from build123d import *
from build123d.topology import SkipClean

# Parameters (mm, degrees)
BOSS_EXTRUDE1_DEPTH = 11
SKETCH3_R           = 2.9
SKETCH3_R_2         = 0.5
CUT_EXTRUDE1_DEPTH  = 4
SKETCH4_W           = 15.75
SKETCH4_H           = 9.4
BOSS_EXTRUDE2_DEPTH = 1
SKETCH5_W           = 15.75
SKETCH5_H           = 9.4
SKETCH5_R           = 1.85
SKETCH5_R_2         = 2.8
CUT_EXTRUDE2_DEPTH  = 1
SKETCH6_W           = 15.75
SKETCH6_H           = 9.4
BOSS_EXTRUDE3_DEPTH = 0.3
CUT_EXTRUDE3_DEPTH  = 0.2
CUT_EXTRUDE4_DEPTH  = 0.1


with BuildPart() as part:
    # Sketch1 → Boss-Extrude1 (new body)
    with BuildSketch(Plane.XY):
        with BuildLine():
            Line((-3, 26.502943725), (-3, -1.102943725))
            ThreePointArc((-3, -1.102943725), (-2.908655439, -1.562163844), (-2.648528137, -1.951471863))
            Line((-2.648528137, -1.951471863), (-2.151471863, -2.448528137))
            ThreePointArc((-2.151471863, -2.448528137), (-1.762163844, -2.708655439), (-1.302943725, -2.8))
            Line((-1.302943725, -2.8), (10.002943725, -2.8))
            ThreePointArc((10.002943725, -2.8), (10.462163844, -2.708655439), (10.851471863, -2.448528137))
            Line((10.851471863, -2.448528137), (16.648528137, 3.348528137))
            ThreePointArc((16.648528137, 3.348528137), (16.908655439, 3.737836156), (17, 4.197056275))
            Line((17, 4.197056275), (17, 27))
            ThreePointArc((17, 27), (16.648528137, 27.848528137), (15.8, 28.2))
            Line((15.8, 28.2), (-1.302943725, 28.2))
            ThreePointArc((-1.302943725, 28.2), (-1.762163844, 28.108655439), (-2.151471863, 27.848528137))
            Line((-2.151471863, 27.848528137), (-2.648528137, 27.351471863))
            ThreePointArc((-2.648528137, 27.351471863), (-2.908655439, 26.962163844), (-3, 26.502943725))
        make_face()
    extrude(amount=-BOSS_EXTRUDE1_DEPTH)

    # Sketch2 → Revolve1 (revolve)
    with BuildSketch(Plane.XY.offset(-5.5), mode=Mode.PRIVATE) as revolve1_sk:
        with BuildLine():
            Line((12, 4.7), (16.899094141, 4.7))
            Line((16.899094141, 4.7), (15.897307991, -4.831358539))
            ThreePointArc((15.897307991, -4.831358539), (15.799690604, -5.022943448), (15.598951422, -5.1))
            Line((15.598951422, -5.1), (15.45, -5.1))
            Line((15.45, -5.1), (15.45, -6.1))
            Line((15.45, -6.1), (16, -6.1))
            Line((16, -6.1), (16, -10.1))
            Line((16, -10.1), (15.25, -10.1))
            Line((15.25, -10.1), (15.25, -11.6))
            Line((15.25, -11.6), (15.45, -11.6))
            Line((15.45, -11.6), (15.45, -12.1))
            Line((15.45, -12.1), (15.25, -13.1))
            Line((15.25, -13.1), (12, -13.1))
            Line((12, -13.1), (12, 4.7))
        make_face()
    revolve(revolve1_sk.sketch.rotate(Axis((12, -13.1, -5.5), (0, 1, 0)), 270), axis=Axis((12, -13.1, -5.5), (0, 1, 0)))

    # Sketch3 → Cut-Extrude1 (cut)
    with BuildSketch(Plane(origin=(0, -9.3, 0), x_dir=(1, 0, 0), z_dir=(0, 1, 0))):
        with Locations(Location((12, 5.5, 0), (0, 0, 270))):
            Circle(SKETCH3_R)
        with Locations(Location((13.41577974, 4.471375808, 0), (0, 0, 270))):
            Circle(SKETCH3_R_2, mode=Mode.SUBTRACT)
        with Locations(Location((13.41577974, 6.528624192, 0), (0, 0, 270))):
            Circle(SKETCH3_R_2, mode=Mode.SUBTRACT)
        with Locations(Location((11.45922026, 3.835651096, 0), (0, 0, 270))):
            Circle(SKETCH3_R_2, mode=Mode.SUBTRACT)
        with Locations(Location((11.45922026, 7.164348904, 0), (0, 0, 270))):
            Circle(SKETCH3_R_2, mode=Mode.SUBTRACT)
    extrude(amount=-CUT_EXTRUDE1_DEPTH, mode=Mode.SUBTRACT)

    # Sketch4 → Boss-Extrude2 (add)
    with BuildSketch(Plane(origin=(0, 28.2, 0), x_dir=(1, 0, 0), z_dir=(0, 1, 0))):
        with Locations((8.075, 5.5)):
            Rectangle(SKETCH4_W, SKETCH4_H)
        Polygon((11.656497116, 4.356497116), (12.529289322, 4.356497116), (12.305025253, 4.580761184), (13.789949494, 6.065685425), (13.365685425, 6.489949494), (11.880761184, 5.005025253), (11.656497116, 5.229289322), align=None, mode=Mode.SUBTRACT)
        Polygon((5.85, 5.9), (5.85, 5.1), (7.35, 5.1), (7.35, 3.6), (8.15, 3.6), (8.15, 5.1), (9.65, 5.1), (9.65, 5.9), (8.15, 5.9), (8.15, 7.4), (7.35, 7.4), (7.35, 5.9), align=None, mode=Mode.SUBTRACT)
    extrude(amount=BOSS_EXTRUDE2_DEPTH)

    # Sketch5 → Cut-Extrude2 (cut)
    with BuildSketch(Plane(origin=(0, 28.2, 0), x_dir=(1, 0, 0), z_dir=(0, 1, 0))):
        with Locations((8.075, 5.5)):
            Rectangle(SKETCH5_W, SKETCH5_H)
        with Locations(Location((12.8, 5.5, 0), (0, 0, 270))):
            Circle(SKETCH5_R, mode=Mode.SUBTRACT)
        with Locations(Location((7.75, 5.5, 0), (0, 0, 270))):
            Circle(SKETCH5_R_2, mode=Mode.SUBTRACT)
    extrude(amount=CUT_EXTRUDE2_DEPTH, mode=Mode.SUBTRACT)

    # Sketch6 → Boss-Extrude3 (add)
    with BuildSketch(Plane(origin=(0, 28.2, 0), x_dir=(1, 0, 0), z_dir=(0, 1, 0))):
        with Locations((8.075, 5.5)):
            Rectangle(SKETCH6_W, SKETCH6_H)
    extrude(amount=BOSS_EXTRUDE3_DEPTH)

    # Sketch7 → Revolve2 (revolve)
    with SkipClean():  # the faces are left unmerged after this step: merging them gives an invalid solid
        with BuildSketch(Plane(origin=(3.1, 0, 0), x_dir=(0, 0, -1), z_dir=(1, 0, 0))):
            with BuildLine():
                Line((8.85, 28), (5.75, 28))
                ThreePointArc((5.75, 28), (7.3, 29.55), (8.85, 28))
            make_face()
        revolve(axis=Axis((3.1, 28, -8.85), (0, 0, 1)))

    # Sketch8 → Cut-Extrude3 (cut)
    with SkipClean():  # the faces are left unmerged after this step: merging them gives an invalid solid
        with BuildSketch(Plane(origin=(-2.8, 0, 0), x_dir=(0, 0, -1), z_dir=(1, 0, 0))):
            with BuildLine():
                Line((1.425, 19.925), (1.425, 2.675))
                ThreePointArc((1.425, 2.675), (1.659314575, 2.109314575), (2.225, 1.875))
                Line((2.225, 1.875), (8.775, 1.875))
                ThreePointArc((8.775, 1.875), (9.340685425, 2.109314575), (9.575, 2.675))
                Line((9.575, 2.675), (9.575, 19.925))
                ThreePointArc((9.575, 19.925), (9.340685425, 20.490685425), (8.775, 20.725))
                Line((8.775, 20.725), (2.225, 20.725))
                ThreePointArc((2.225, 20.725), (1.659314575, 20.490685425), (1.425, 19.925))
            make_face()
        extrude(amount=-CUT_EXTRUDE3_DEPTH, mode=Mode.SUBTRACT)

    # Sketch9 → Cut-Extrude4 (cut)
    with SkipClean():  # the faces are left unmerged after this step: merging them gives an invalid solid
        with BuildSketch(Plane.XY.offset(-11)):
            with BuildLine():
                Line((4.4, 0.2), (9.091673888, 0.2))
                ThreePointArc((9.091673888, 0.2), (9.244747261, 0.230448187), (9.3745166, 0.317157288))
                Line((9.3745166, 0.317157288), (13.882842712, 4.8254834))
                ThreePointArc((13.882842712, 4.8254834), (13.969551813, 4.955252739), (14, 5.108326112))
                Line((14, 5.108326112), (14, 24.8))
                ThreePointArc((14, 24.8), (13.882842712, 25.082842712), (13.6, 25.2))
                Line((13.6, 25.2), (4.4, 25.2))
                ThreePointArc((4.4, 25.2), (4.117157288, 25.082842712), (4, 24.8))
                Line((4, 24.8), (4, 0.6))
                ThreePointArc((4, 0.6), (4.117157288, 0.317157288), (4.4, 0.2))
            make_face()
        extrude(amount=CUT_EXTRUDE4_DEPTH, mode=Mode.SUBTRACT)

    # Sketch10 → Cut-Revolve1 (revolve, cut)
    with SkipClean():  # the faces are left unmerged after this step: merging them gives an invalid solid
        with BuildSketch(Plane(origin=(0, 0, 0), x_dir=(0, 0, -1), z_dir=(1, 0, 0)), mode=Mode.PRIVATE) as cut_revolve1_sk:
            Polygon((0, 0), (0, 1.5), (0.2705, 1.2295), (10.7295, 1.2295), (11, 1.5), (11, 0), align=None)
        revolve(cut_revolve1_sk.sketch.rotate(Axis((0, 0, -11), (0, 0, 1)), 270), axis=Axis((0, 0, -11), (0, 0, 1)), mode=Mode.SUBTRACT)

    # Sketch11 → Cut-Revolve2 (revolve, cut)
    with SkipClean():  # the faces are left unmerged after this step: merging them gives an invalid solid
        with BuildSketch(Plane(origin=(0, 0, 0), x_dir=(0, 0, -1), z_dir=(1, 0, 0)), mode=Mode.PRIVATE) as cut_revolve2_sk:
            Polygon((0, 25.4), (0, 26.9), (0.2705, 26.6295), (10.7295, 26.6295), (11, 26.9), (11, 25.4), align=None)
        revolve(cut_revolve2_sk.sketch.rotate(Axis((0, 25.4, -11), (0, 0, 1)), 270), axis=Axis((0, 25.4, -11), (0, 0, 1)), mode=Mode.SUBTRACT)

    # Sketch12 → Revolve3 (revolve)
    with SkipClean():  # the faces are left unmerged after this step: merging them gives an invalid solid
        with BuildSketch(Plane(origin=(3.1, 0, 0), x_dir=(0, 0, -1), z_dir=(1, 0, 0))):
            with BuildLine():
                Line((5.15, 28), (2.05, 28))
                ThreePointArc((2.05, 28), (3.6, 29.55), (5.15, 28))
            make_face()
        revolve(axis=Axis((3.1, 28, -5.15), (0, 0, 1)))


solid = part.part
For this review, take the finished solid that the model builds, in its own axes (mm). A direction names the side the tool comes from. Round coordinates to 2 decimals unless told otherwise and drop trailing zeros. Write each question's results on one line, items separated by ' | '. Start each with the question number.
1. Draft analysis for pull direction X (two halves, no side actions). For faces 1 (the face through (13.44, -11.17, -4.97)), 2 (the face through (8.3, 29.2, -4.9)), 3 (the face through (5.266, 28.845, -4.208)), 4 (the face through (-2.91, -1.56, -5.42)), state which applies: pulls with the +X half, pulls with the -X half, needs draft (parallel to the pull), parting line crosses it, or undercut.
2. Clearance check with flat-ended pins moving along their axes: pin 1 Ø1.5 at (y, z) = (16, -4.5) entering from -X; pin 2 Ø5 at (y, z) = (-2.5, -7) entering from -X; pin 3 Ø0.8 at (y, z) = (29, -5) entering from +X; pin 4 Ø5.5 at (x, z) = (12.5, -4) entering from +Y. State where each tip first meets the part, or that it passes through.
3. Tool access review of faces 5 (the face through (10.46, -2.71, -10.25)), 6 (the face through (14, -11.2, -7.6)), 7 (the face through (13.4, -13.1, -6.5)), 8 (the face through (9, 13, -10.9)), 9 (the face through (9.901, -5.607, -8.238)): name each direction out of +Z, -Z, +X, -X, +Y, -Y from which nothing blocks a thin tool from reaching the whole face with its end or side.
4. To check wall thickness, follow L1, parallel to Y at x = 0, z = -7.25; L2, parallel to Y at x = 12, z = -1.75; L3, parallel to X at y = -11, z = -4.5. State the ranges of each line that lie inside material, in increasing order. Write a range as [from, to].
Output values:
1) face 1: undercut | face 2: needs draft | face 3: undercut | face 4: pulls with the -X half
2) pin 1: x = -2.8 | pin 2: x = -3 | pin 3: x = 14.65 | pin 4: y = 29.2
3) face 5: -Z, -Y | face 6: -Y | face 7: +Z, -Z, +X, -X, -Y | face 8: -Z | face 9: none
4) L1: [-2.8, -1.23], [1.23, 24.17], [26.63, 28.2] | L2: [-10.1, -6.1], [-5.06, 28.5] | L3: [8.91, 9.28], [12.92, 13.91], [14.72, 15.09]
